Geometry check sheet. Reference: drawing and pictorial views, mm from the part's lowest x, y, z. A direction names the side the tool comes from. Give positions to 0.01 mm unless a question says otherwise; leave off trailing zeros. Write each loop counter-clockwise with the first axis right and the second up, starting at its lowest first coordinate (ties: lowest second). Pieces come first, ordered by that corner, then holes. Notation, with made-up numbers: M 40.25,47 L 89.25,47 A22 ccw 89.25,64 Z; hole C 19,47 d4. An arc over 180 degrees is marked long. Answer as a JSON object with one key per item and string values.
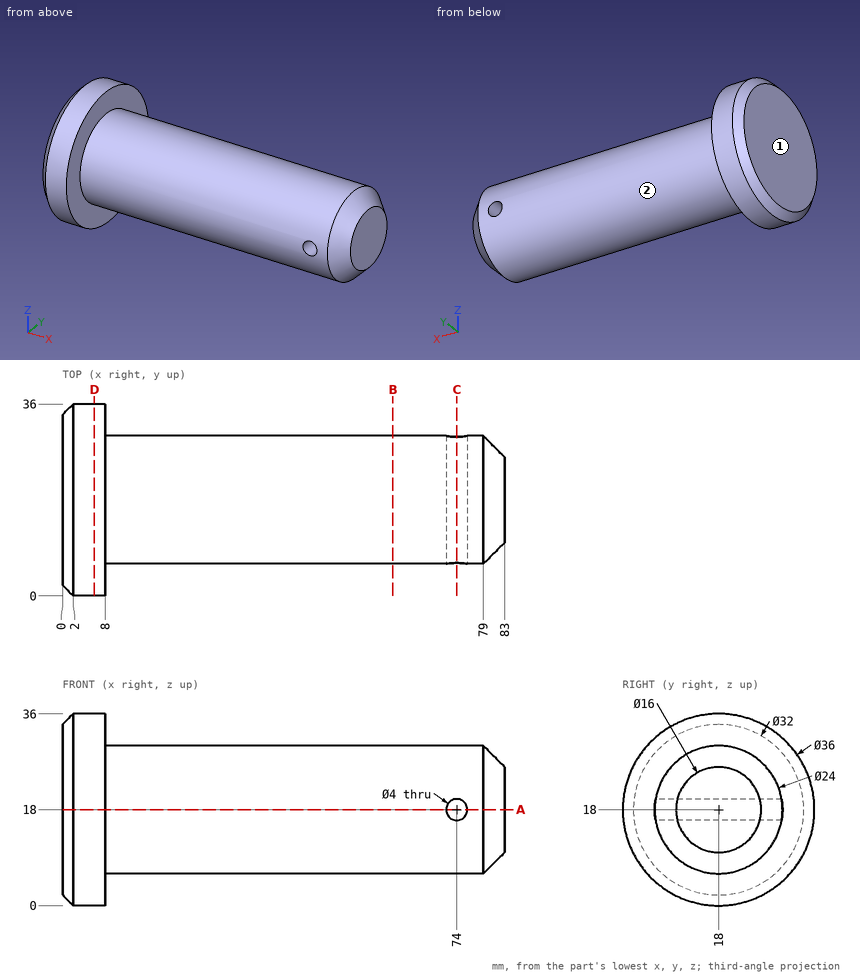
1) Thickness scan on L1, parallel to X at y = 19.75, z = 18; L2, parallel to Z at x = 74, y = 22.5; L3, parallel to X at y = 12, z = 5.5. Record the ranges inside material, lowest first.
Completed:
{"L1": "x = 0 to 72, 76 to 83", "L2": "z = 6.88 to 16, 20 to 29.12", "L3": "x = 0 to 8"}
2) Section check B-B on x = 62. Record the boundary of the cut face in (y, z), and give its area (3 significant figures).
Completed:
{"outline": "C 18,18 d24", "area": "452 mm2"}
3) Section check D-D on x = 6. Record the boundary of the cut face in (y, z), and give its area (3 significant figures).
Completed:
{"outline": "C 18,18 d36", "area": "1,020 mm2"}
4) Go/stop test with flat-tipped pins: pin 1 (5 mm diameter, centred on x = 74, z = 18, fed in from -Y); pin 2 (2 mm diameter, centred on x = 12, y = 8.5, fed in from +Z); pin 3 (4 mm diameter, centred on x = 25, z = 10, fed in from +Y). Record where each tip stops, or that it passes through.
Completed:
{"pin 1": "stops at y = 6", "pin 2": "stops at z = 26.47", "pin 3": "stops at y = 28.39"}
5) Section check A-A on z = 18. Record the boundary of the cut face in (x, y), and give its area (3 significant figures).
Completed:
{"outline": "M 0,2 L 2,0 L 8,0 L 8,6 L 72,6 L 72,30 L 8,30 L 8,36 L 2,36 L 0,34 Z; M 76,6 L 79,6 L 83,10 L 83,26 L 79,30 L 76,30 Z", "area": "1,970 mm2"}
6) Section check C-C on x = 74. Record the boundary of the cut face in (y, z), and give its area (3 significant figures).
Completed:
{"outline": "M 6.17,16 A12 ccw 29.83,16 Z; M 6.17,20 L 29.83,20 A12 ccw Z", "area": "357 mm2"}
7) Access from +Z, -Z, +X, -X, +Y, -Y to the whole of each face (thin tool, end or side, straight path). Record for the marked faces 1 and 2.
Completed:
{"face 1": "+Z, -Z, -X, +Y, -Y", "face 2": "+X"}
